Read the model definition and answer for the solid it produces. Units are mm, in the model's axes. Face numbers are marked on the shaded views. A direction names the side the tool comes from. Give positions to 0.01 mm unless a question says otherwise; leave off trailing zeros. Order: outer loops, then holes, each group sorted by start corner. A loop starts at its lowest first (then second) coordinate and runs counter-clockwise, first axis right, second up. Notation, with made-up numbers: (88, -20) - (121, -20) arc R18 ccw to (121, -7) - close; hole circle Ø10 at (89, -6.75). An arc over 180 degrees is marked (long way). Return JSON: item names as keys, results as strings.
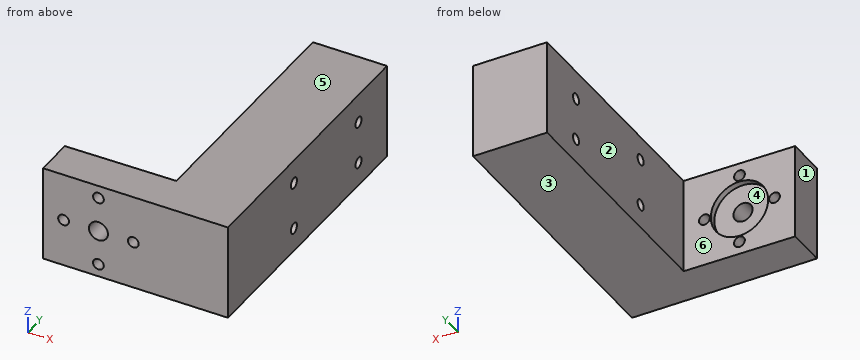
```python
from build123d import *

# Parameters (mm, degrees)
BOSS_EXTRUDE1_DEPTH = 30
CUT_EXTRUDE1_REACH  = 103.41
SKETCH2_R           = 3
SKETCH2_R_2         = 1.7
SKETCH3_R           = 9
CUT_EXTRUDE2_DEPTH  = 2
CUT_EXTRUDE3_REACH  = 102.783
SKETCH4_R           = 1.7


with BuildPart() as part:
    # Sketch1 → Boss-Extrude1 (new body)
    with BuildSketch(Plane.XY):
        Polygon((0, 0), (58.399287612, -0.629459459), (58.399287612, 89.370540541), (35, 89.622750859), (35, 12.334557553), (0, 12.334557553), align=None)
    extrude(amount=BOSS_EXTRUDE1_DEPTH)

    # Cut-Extrude1: up to this plane
    cut_extrude1_end = Plane(origin=(0, 0, 30), z_dir=(0.010777920827534888, 0.9999419165244726, 0))
    # Sketch2 → Cut-Extrude1 (cut, up to the surface)
    with BuildSketch(Plane(origin=(0, 12.334557553, 0), x_dir=(1, 0, 0), z_dir=(0, 1, 0)), mode=Mode.PRIVATE) as cut_extrude1_sk1:
        with Locations(Location((17.5, -15, 0), (0, 0, 180))):
            Circle(SKETCH2_R)
    cut_extrude1_tool1 = split(extrude(cut_extrude1_sk1.sketch, amount=-CUT_EXTRUDE1_REACH, mode=Mode.PRIVATE), bisect_by=cut_extrude1_end, keep=Keep.BOTH, mode=Mode.PRIVATE)
    add(cut_extrude1_tool1.solids().sort_by_distance((17.5, 12.334558, 15))[0], mode=Mode.SUBTRACT)
    # Sketch2 → Cut-Extrude1 (cut, up to the surface)
    with BuildSketch(Plane(origin=(0, 12.334557553, 0), x_dir=(1, 0, 0), z_dir=(0, 1, 0)), mode=Mode.PRIVATE) as cut_extrude1_sk2:
        with Locations(Location((6.5, -15, 0), (0, 0, 180))):
            Circle(SKETCH2_R_2)
    cut_extrude1_tool2 = split(extrude(cut_extrude1_sk2.sketch, amount=-CUT_EXTRUDE1_REACH, mode=Mode.PRIVATE), bisect_by=cut_extrude1_end, keep=Keep.BOTH, mode=Mode.PRIVATE)
    add(cut_extrude1_tool2.solids().sort_by_distance((6.5, 12.334558, 15))[0], mode=Mode.SUBTRACT)
    # Sketch2 → Cut-Extrude1 (cut, up to the surface)
    with BuildSketch(Plane(origin=(0, 12.334557553, 0), x_dir=(1, 0, 0), z_dir=(0, 1, 0)), mode=Mode.PRIVATE) as cut_extrude1_sk3:
        with Locations(Location((17.5, -4, 0), (0, 0, 180))):
            Circle(SKETCH2_R_2)
    cut_extrude1_tool3 = split(extrude(cut_extrude1_sk3.sketch, amount=-CUT_EXTRUDE1_REACH, mode=Mode.PRIVATE), bisect_by=cut_extrude1_end, keep=Keep.BOTH, mode=Mode.PRIVATE)
    add(cut_extrude1_tool3.solids().sort_by_distance((17.5, 12.334558, 4))[0], mode=Mode.SUBTRACT)
    # Sketch2 → Cut-Extrude1 (cut, up to the surface)
    with BuildSketch(Plane(origin=(0, 12.334557553, 0), x_dir=(1, 0, 0), z_dir=(0, 1, 0)), mode=Mode.PRIVATE) as cut_extrude1_sk4:
        with Locations(Location((28.5, -15, 0), (0, 0, 180))):
            Circle(SKETCH2_R_2)
    cut_extrude1_tool4 = split(extrude(cut_extrude1_sk4.sketch, amount=-CUT_EXTRUDE1_REACH, mode=Mode.PRIVATE), bisect_by=cut_extrude1_end, keep=Keep.BOTH, mode=Mode.PRIVATE)
    add(cut_extrude1_tool4.solids().sort_by_distance((28.5, 12.334558, 15))[0], mode=Mode.SUBTRACT)
    # Sketch2 → Cut-Extrude1 (cut, up to the surface)
    with BuildSketch(Plane(origin=(0, 12.334557553, 0), x_dir=(1, 0, 0), z_dir=(0, 1, 0)), mode=Mode.PRIVATE) as cut_extrude1_sk5:
        with Locations(Location((17.5, -26, 0), (0, 0, 180))):
            Circle(SKETCH2_R_2)
    cut_extrude1_tool5 = split(extrude(cut_extrude1_sk5.sketch, amount=-CUT_EXTRUDE1_REACH, mode=Mode.PRIVATE), bisect_by=cut_extrude1_end, keep=Keep.BOTH, mode=Mode.PRIVATE)
    add(cut_extrude1_tool5.solids().sort_by_distance((17.5, 12.334558, 26))[0], mode=Mode.SUBTRACT)

    # Sketch3 → Cut-Extrude2 (cut)
    with BuildSketch(Plane(origin=(0, 12.334557553, 0), x_dir=(1, 0, 0), z_dir=(0, 1, 0))):
        with Locations(Location((17.5, -15, 0), (0, 0, 180))):
            Circle(SKETCH3_R)
    extrude(amount=-CUT_EXTRUDE2_DEPTH, mode=Mode.SUBTRACT)

    # Sketch4 → Cut-Extrude3 (cut, up to next)
    with BuildSketch(Plane.ZY.offset(-35), mode=Mode.PRIVATE) as cut_extrude3_sk1:
        with Locations(Location((22.5, 36.700540541, 0), (0, 0, 270))):
            Circle(SKETCH4_R)
    cut_extrude3_tool1 = extrude(cut_extrude3_sk1.sketch, amount=-CUT_EXTRUDE3_REACH, mode=Mode.PRIVATE) & part.part
    # Sketch4 → Cut-Extrude3 (cut, up to next)
    with BuildSketch(Plane.ZY.offset(-35), mode=Mode.PRIVATE) as cut_extrude3_sk2:
        with Locations(Location((7.5, 36.700540541, 0), (0, 0, 270))):
            Circle(SKETCH4_R)
    cut_extrude3_tool2 = extrude(cut_extrude3_sk2.sketch, amount=-CUT_EXTRUDE3_REACH, mode=Mode.PRIVATE) & part.part
    # Sketch4 → Cut-Extrude3 (cut, up to next)
    with BuildSketch(Plane.ZY.offset(-35), mode=Mode.PRIVATE) as cut_extrude3_sk3:
        with Locations(Location((7.5, 73.270540541, 0), (0, 0, 270))):
            Circle(SKETCH4_R)
    cut_extrude3_tool3 = extrude(cut_extrude3_sk3.sketch, amount=-CUT_EXTRUDE3_REACH, mode=Mode.PRIVATE) & part.part
    # Sketch4 → Cut-Extrude3 (cut, up to next)
    with BuildSketch(Plane.ZY.offset(-35), mode=Mode.PRIVATE) as cut_extrude3_sk4:
        with Locations(Location((20.905297153, 73.270540541, 0), (0, 0, 270))):
            Circle(SKETCH4_R)
    cut_extrude3_tool4 = extrude(cut_extrude3_sk4.sketch, amount=-CUT_EXTRUDE3_REACH, mode=Mode.PRIVATE) & part.part
    add(cut_extrude3_tool1.solids().sort_by_distance((35, 36.700541, 22.5))[0], mode=Mode.SUBTRACT)
    add(cut_extrude3_tool2.solids().sort_by_distance((35, 36.700541, 7.5))[0], mode=Mode.SUBTRACT)
    add(cut_extrude3_tool3.solids().sort_by_distance((35, 73.270541, 7.5))[0], mode=Mode.SUBTRACT)
    add(cut_extrude3_tool4.solids().sort_by_distance((35, 73.270541, 20.905297))[0], mode=Mode.SUBTRACT)


solid = part.part
```
Q1. Determine the mould class of the marked faces 3, 4, 5 and 6 for opening direction Z: released by +Z, released by -Z, zero draft, split by the parting line, or undercut.
Values:
{"face 3": "released by -Z", "face 4": "undercut", "face 5": "released by +Z", "face 6": "zero draft"}
Q2. Given pin 1 (14.5 mm diameter, centred on x = 14.5, z = 19, fed in from +Y); pin 2 (5.5 mm diameter, centred on y = 73.27, z = 7.5, fed in from -X); pin 3 (14.5 mm diameter, centred on x = 17.5, z = 15, fed in from -Y), each flat-ended and moving along its own axis, determine where each tip first touches the part or whether it passes through.
Values:
{"pin 1": "stops at y = 12.33", "pin 2": "stops at x = 35", "pin 3": "stops at y = -0.27"}
Q3. A cutting plane is placed at B-B (z = 15). Write down the section's boundary in (x, y), and give its area (3 significant figures).
Values:
{"outline": "(0, 0) - (4.8, -0.05) - (4.8, 12.33) - (0, 12.33) - close; (8.2, -0.09) - (14.5, -0.16) - (14.5, 10.33) - (8.5, 10.33) - (8.5, 12.33) - (8.2, 12.33) - close; (20.5, -0.22) - (26.8, -0.29) - (26.8, 12.33) - (26.5, 12.33) - (26.5, 10.33) - (20.5, 10.33) - close; (30.2, -0.33) - (58.4, -0.63) - (58.4, 89.37) - (35, 89.62) - (35, 12.33) - (30.2, 12.33) - close", "area": "2,360 mm²"}
Q4. Consider L1, parallel to Z at x = 17.5, y = 7; L2, parallel to Z at x = 6.5, y = 2.75; L3, parallel to X at y = 16, z = 16.25. Determine where each line is inside the solid, lowest interval first.
Values:
{"L1": "z = 0 to 2.3, 5.7 to 12, 18 to 24.3, 27.7 to 30", "L2": "z = 0 to 13.3, 16.7 to 30", "L3": "x = 35 to 58.4"}
Q5. For the marked faces 1 and 2, determine the directions among +Z, -Z, +X, -X, +Y, -Y from which every point of the face is accessible in a straight line to the end or side of a thin tool.
Values:
{"face 1": "+Z, -Z, -X, +Y, -Y", "face 2": "+Z, -Z, -X, +Y"}
Q6. A cutting plane is placed at C-C (y = 36). Write down the section's boundary in (x, z).
Values:
{"outline": "(35, 0) - (58.4, 0) - (58.4, 5.95) - (35, 5.95) - close; (35, 9.05) - (58.4, 9.05) - (58.4, 20.95) - (35, 20.95) - close; (35, 24.05) - (58.4, 24.05) - (58.4, 30) - (35, 30) - close"}
Q7. A cutting plane is placed at D-D (x = 51.5). Write down the section's boundary in (y, z), and give its area (3 significant figures).
Values:
{"outline": "(-0.56, 0) - (89.44, 0) - (89.44, 30) - (-0.56, 30) - close; hole circle Ø3.4 at (36.7, 7.5); hole circle Ø3.4 at (36.7, 22.5); hole circle Ø3.4 at (73.27, 7.5); hole circle Ø3.4 at (73.27, 20.91)", "area": "2,660 mm²"}
Q8. A cutting plane is placed at A-A (x = 6.5). Write down the section's boundary in (y, z).
Values:
{"outline": "(-0.07, 0) - (12.33, 0) - (12.33, 13.3) - (-0.07, 13.3) - close; (-0.07, 16.7) - (12.33, 16.7) - (12.33, 30) - (-0.07, 30) - close"}
